Can you work these out from the drawing? Everything is in mm from the part's minimum corner. A direction names the side the tool comes from. Round coordinates to 2 decimals unless told otherwise and drop trailing zeros. Loops run counter-clockwise (first coordinate to the right, second up) from the corner with the lowest first, then second, coordinate; pieces in that order, holes last. Notation, with made-up numbers: M -36,3.25 L -31,3.25 A28 ccw -31,22.25 Z; hole C 38.25,21.25 d4. An arc over 180 degrees is marked long. One line per question, with ' | ' between items. Start each with the question number.
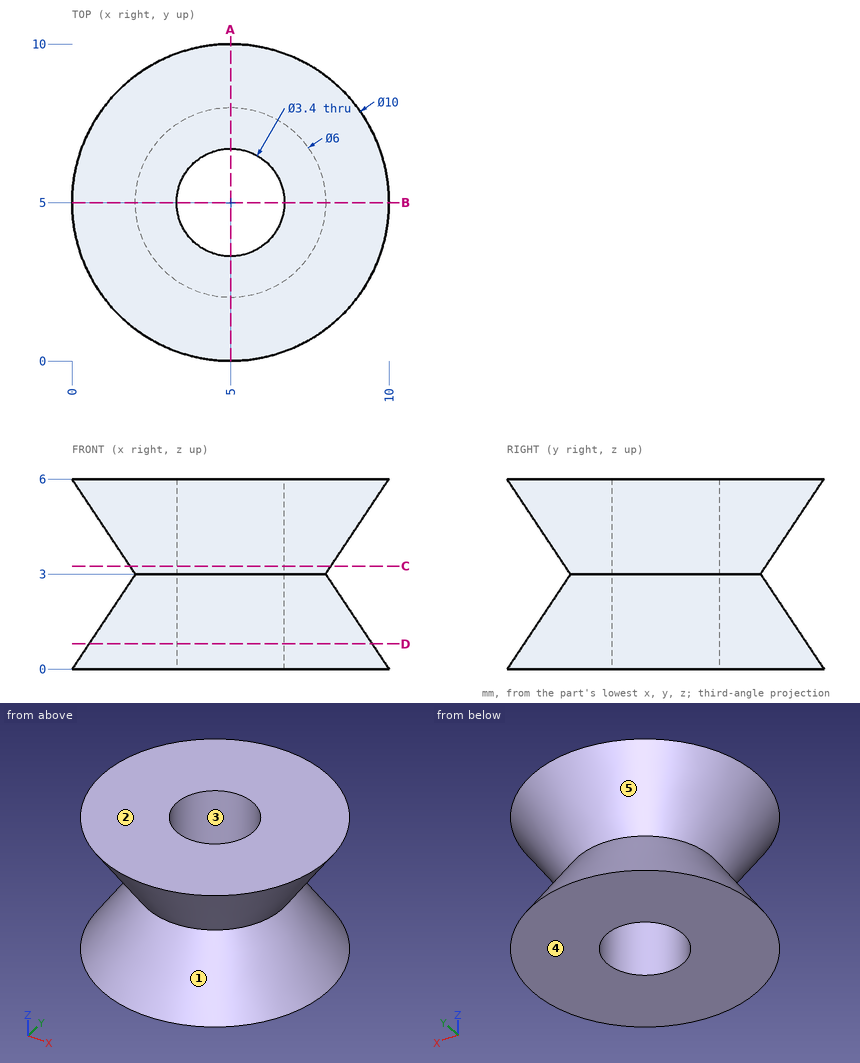
1) Imagine slicing it at D-D (z = 0.8). Write out the boundary of the cut face in (x, y).
2) Imagine slicing it at C-C (z = 3.25). Write out the boundary of the cut face in (x, y).
3) I'm going to push flat-ended pins straight in: pin 1 Ø1 at (x, y) = (8.5, 2.5) entering from -Z; pin 2 Ø3 at (x, y) = (5, 5) entering from -Z; pin 3 Ø1 at (y, z) = (6.5, 1) entering from +X; pin 4 Ø1.5 at (x, z) = (3.5, 5) entering from -Y. Where does each tip first touch, or does it pass through?
4) For the marked faces 4 and 5, which set-ups out of +Z, -Z, +X, -X, +Y, -Y let a thin tool reach every point of the face, with its end or its side?
5) Please list where these lines run through material, in increasing order: L1, parallel to X at y = 6.5, z = 3.5; L2, parallel to Z at x = 1.75, y = 7.5; L3, parallel to Z at x = 4.75, y = 9. Write a range as from..to.
6) Imagine slicing it at A-A (x = 5). Write out the boundary of the cut face in (y, z).
7) We'd pull the mould along Y, two halves only. Please class the marked faces 1, 2 and 3: pulls with the +Y half, pulls with the -Y half, needs draft (parallel to the pull), parting line crosses it, or undercut.
Results are:
1) outline: C 5,5 d8.93; hole C 5,5 d3.4
2) outline: C 5,5 d6.33; hole C 5,5 d3.4
3) pin 1: z = 0 | pin 2: through | pin 3: x = 9.45 | pin 4: y = 0.36
4) face 4: -Z, +X, -X, +Y, -Y | face 5: none
5) L1: 2.02..4.2, 5.8..7.98 | L2: 0..1.35, 4.65..6 | L3: 0..1.49, 4.51..6
6) outline: M 0,0 L 3.3,0 L 3.3,6 L 0,6 L 2,3 Z; M 6.7,0 L 10,0 L 8,3 L 10,6 L 6.7,6 Z
7) face 1: parting line crosses it | face 2: needs draft | face 3: undercut
